Input: part model. Units: mm. Frame: model coordinates. A direction names the side the tool comes from. Coordinates: 2 decimals unless noted, no trailing zeros. Loops run counter-clockwise (first coordinate to the right, second up) from the corner with the lowest first, then second, coordinate; pieces in that order, holes last. Notation, with made-up numbers: (-10, -22) - (2, -22) arc R25 cw to (2, -9) - close; hole circle Ø4 at (43, 41.25). An arc over 180 degrees is marked (long way). Use a Markdown table: item, result. Add a question column.
1. Section query B-B on z = 7. Return the cut outline in (x, y), then the cut area to 3 significant figures.
2. Section query D-D on z = 18. Return the cut outline in (x, y), then the cut area to 3 significant figures.
3. Draft query along Y for faces 1 (the face through (41, -15.5, 11)), 2 (the face through (-13, -56, 17)), 3 (the face through (43, -16, 16)). Return one class per face: released by +Y, released by -Y, zero draft, split by the parting line, or undercut.
4. Ray query, L1, parallel to Y at x = 44, z = 2.15; L2, parallel to Z at x = -3.5, y = 13; L3, parallel to X at y = -50.5, z = 25.5. Return the intervals inside material, ascending. Write a range as [from, to].
5. Contact query for flat-ended pins moving along their axis: P1, Ø9.5, axis at x = -31, z = 18.5, coming from the +Y side; P2, Ø8, axis at x = 39, z = 14, coming from the -Y side; P3, Ø1.6, axis at x = 32.5, y = -5.5, coming from the +Z side; P4, Ø6, axis at y = 22, z = 9, coming from the -X side. Output: stop coordinate, or through.
6. Access query for faces 4 (the face through (40, 17.5, 10)), 5 (the face through (40, -17.5, 10)), 6 (the face through (52, -1.4, 4.6)), 7 (the face through (34, 0, 13)), 8 (the face through (-49.197, -36, 19)). Directions: +Z, -Z, +X, -X, +Y, -Y. A direction counts if a zero-diameter tool reaches every point of the face in a straight line with its end or side. Return the directions, or none.
7. Section query A-A on x = -44. Return the cut outline in (y, z).
8. Section query C-C on y = 4.5. Return the cut outline in (x, z), then the cut area to 3 significant figures.
```python
from build123d import *

# Parameters (mm, degrees)
SKETCH1_W           = 112
SKETCH1_H           = 112
BOSS_EXTRUDE1_DEPTH = 3
SKETCH2_W           = 50
SKETCH2_H           = 40
BOSS_EXTRUDE2_DEPTH = 32
CUT_EXTRUDE1_REACH  = 5
SKETCH3_R           = 1.5
SKETCH4_W           = 20
SKETCH4_H           = 35
BOSS_EXTRUDE3_DEPTH = 18
SKETCH5_W           = 18
SKETCH5_H           = 31
CUT_EXTRUDE2_DEPTH  = 16
CUT_EXTRUDE3_DEPTH  = 74.5


with BuildPart() as part:
    # Sketch1 → Boss-Extrude1 (new body)
    with BuildSketch(Plane.XY):
        Rectangle(SKETCH1_W, SKETCH1_H)
    extrude(amount=BOSS_EXTRUDE1_DEPTH)

    # Sketch2 → Boss-Extrude2 (add)
    with BuildSketch(Plane.XY.offset(3)):
        with Locations((-24.196765027, -36)):
            Rectangle(SKETCH2_W, SKETCH2_H)
    extrude(amount=BOSS_EXTRUDE2_DEPTH)

    # Sketch3 → Cut-Extrude1 (cut, up to next)
    with BuildSketch(Plane.XY.offset(3), mode=Mode.PRIVATE) as cut_extrude1_sk1:
        with Locations((-44, 46)):
            Circle(SKETCH3_R)
    cut_extrude1_tool1 = extrude(cut_extrude1_sk1.sketch, amount=-CUT_EXTRUDE1_REACH, mode=Mode.PRIVATE) & part.part
    add(cut_extrude1_tool1.solids().sort_by_distance((-44, 46, 3))[0], mode=Mode.SUBTRACT)
    # Sketch3 → Cut-Extrude1 (cut, up to next)
    with BuildSketch(Plane.XY.offset(3), mode=Mode.PRIVATE) as cut_extrude1_sk2:
        with Locations((44, 46)):
            Circle(SKETCH3_R)
    cut_extrude1_tool2 = extrude(cut_extrude1_sk2.sketch, amount=-CUT_EXTRUDE1_REACH, mode=Mode.PRIVATE) & part.part
    add(cut_extrude1_tool2.solids().sort_by_distance((44, 46, 3))[0], mode=Mode.SUBTRACT)
    # Sketch3 → Cut-Extrude1 (cut, up to next)
    with BuildSketch(Plane.XY.offset(3), mode=Mode.PRIVATE) as cut_extrude1_sk3:
        with Locations((6.803234973, -46)):
            Circle(SKETCH3_R)
    cut_extrude1_tool3 = extrude(cut_extrude1_sk3.sketch, amount=-CUT_EXTRUDE1_REACH, mode=Mode.PRIVATE) & part.part
    add(cut_extrude1_tool3.solids().sort_by_distance((6.803235, -46, 3))[0], mode=Mode.SUBTRACT)

    # Sketch4 → Boss-Extrude3 (add)
    with BuildSketch(Plane.XY.offset(3)):
        with Locations((42, 0)):
            Rectangle(SKETCH4_W, SKETCH4_H)
    extrude(amount=BOSS_EXTRUDE3_DEPTH)

    # Sketch5 → Cut-Extrude2 (cut)
    with BuildSketch(Plane.XY.offset(21)):
        with Locations((43, 0)):
            Rectangle(SKETCH5_W, SKETCH5_H)
    extrude(amount=-CUT_EXTRUDE2_DEPTH, mode=Mode.SUBTRACT)

    # Sketch6 → Cut-Extrude3 (cut, through all)
    with BuildSketch(Plane(origin=(0, 17.5, 0), x_dir=(1, 0, 0), z_dir=(0, 1, 0))):
        Polygon((34, -21), (52, -11), (52, -21), align=None)
    extrude(amount=-CUT_EXTRUDE3_DEPTH, mode=Mode.SUBTRACT)


solid = part.part
```
Resolved:
| question | item | result |
|---|---|---|
| 1 | outline | (-49.2, -56) - (0.8, -56) - (0.8, -16) - (-49.2, -16) - close; (32, -17.5) - (52, -17.5) - (52, -15.5) - (34, -15.5) - (34, 15.5) - (52, 15.5) - (52, 17.5) - (32, 17.5) - close |
| 1 | area | 2,140 mm² |
| 2 | outline | (-49.2, -56) - (0.8, -56) - (0.8, -16) - (-49.2, -16) - close; (32, -17.5) - (39.4, -17.5) - (39.4, -15.5) - (34, -15.5) - (34, 15.5) - (39.4, 15.5) - (39.4, 17.5) - (32, 17.5) - close |
| 2 | area | 2,090 mm² |
| 3 | face 1 | undercut |
| 3 | face 2 | released by -Y |
| 3 | face 3 | zero draft |
| 4 | L1 | [-56, 44.5], [47.5, 56] |
| 4 | L2 | [0, 3] |
| 4 | L3 | [-49.2, 0.8] |
| 5 | P1 | y = -16 |
| 5 | P2 | y = -17.5 |
| 5 | P3 | z = 21 |
| 5 | P4 | through |
| 6 | face 4 | +Z, +X, -X, +Y |
| 6 | face 5 | +Z, +X, -Y |
| 6 | face 6 | +Z, +X, +Y, -Y |
| 6 | face 7 | +Z, +X |
| 6 | face 8 | +Z, -X, +Y, -Y |
| 7 | outline | (-56, 0) - (44.5, 0) - (44.5, 3) - (-16, 3) - (-16, 35) - (-56, 35) - close; (47.5, 0) - (56, 0) - (56, 3) - (47.5, 3) - close |
| 8 | outline | (-56, 0) - (56, 0) - (56, 3) - (52, 3) - (52, 5) - (34, 5) - (34, 21) - (32, 21) - (32, 3) - (-56, 3) - close |
| 8 | area | 408 mm² |
